Read the model definition and answer for the solid it produces. Units are mm, in the model's axes. A direction names the side the tool comes from. Coordinates: 2 decimals unless noted, no trailing zeros. Order: outer loops, then holes, each group sorted by start corner. A loop starts at its lowest first (then second) coordinate and runs counter-clockwise, first axis right, second up. Notation, with made-up numbers: M 58,6 L 68,6 A22 ccw 68,32 Z; hole C -39.75,-38.75 d11. An arc over 180 degrees is marked long. Put each result on its own line as item: value.
from build123d import *

# Parameters (mm, degrees)
F0_R         = 56.0284560605
F1_DEPTH     = 56.18732
F2_T         = -2.54
F3_W         = 7.7828075737
F3_H         = 34.1701302677
F4_DEPTH     = 276.60562
F6_R         = 34.5946759053
F7_DEPTH     = 25.4
F8_T         = 2.54
F8_T3_DEPTH  = 39.2501302677
F8_T5_DEPTH  = 12.8628075737
F10_SIZE     = 2.54
F11_W        = 6.7604319192
F11_H        = 35.768898204
F12_DEPTH    = 28.2828
F13_W        = 6.7604319192
F13_H        = 35.768898204
F14_DEPTH    = 6.19419
F15_W        = 35.768898204
F15_H        = 8.6004413581
F16_DEPTH    = 43.51639
F17_W        = 31.8477451801
F17_H        = 4.8072040081
F18_DEPTH    = 48.07886
F19_DEPTH    = 32.39902
F20_R        = 5.08
F21_T1_DEPTH = 61.168898204
F22_R        = 1.27


# Not quite as in the source:
# - a fillet or chamfer that OpenCascade refuses, or shapes differently, is made with other operations: its cross-section is extruded or revolved along the edge and cut away or added
# - a shell that OpenCascade refuses in one call is made with other operations: the cavity is built on its own and cut out


with BuildPart() as f1:
    # F0 (on Top) → F1 (new body)
    with BuildSketch(Plane.XY):
        Circle(F0_R)
    extrude(amount=F1_DEPTH)

    # F2
    f2_openings = [f1.faces().sort_by_distance(p)[0] for p in [
        (0, 0, 0),
    ]]
    offset(amount=F2_T, openings=f2_openings)

    # F3 (on face) → F4 (join)
    with BuildSketch(Plane(origin=(0, 0, 53.64732), x_dir=(1, 0, 0), z_dir=(0, 0, -1))):
        with Locations((0.0409056073, 0.1802544365)):
            Rectangle(F3_W, F3_H)
    extrude(amount=F4_DEPTH)

    # F5: chamfer of 5.08 on 1 edges, made by hand

    # F5_s1 → F5_t2 (revolve, cut)
    with BuildSketch(Plane.XZ):
        Polygon((58.5684560605, 0), (53.4884560605, 5.08), (53.4884560605, 0), align=None)
    revolve(axis=Axis((0, 0, 0), (0, 0, 1)), mode=Mode.SUBTRACT)

    # F6 (on face) → F7 (join)
    with BuildSketch(Plane.XY.offset(56.18732)):
        Circle(F6_R)
    extrude(amount=F7_DEPTH)

    # F8: shell of thickness 2.54, made by hand


with BuildPart() as f8_core1:
    # F8_t2: copy of F1
    add(f1.part)

    # the walls: a layer under each face that stays
    f8_faces = [f8_core1.faces().sort_by_distance(p)[0] for p in [
        (-56.0284560605, 0, 29.36366),
        (-54.7584560605, 0, 3.81),
        (-37.3523040403, -37.3523040403, 56.18732),
        (-53.4884560605, 0, 29.36366),
        (-34.5946759053, 0, 68.88732),
        (-35.658970707, -35.658970707, 53.64732),
        (3.9323093942, -0.1802544365, -84.65549),
        (0.0409056073, 16.9048106974, -84.65549),
        (-3.8504981795, -0.1802544365, -84.65549),
        (0.0409056073, -17.2653195703, -84.65549),
    ]]
    thicken(f8_faces, amount=-F8_T, mode=Mode.SUBTRACT)

    # F8_s4 → F8_t3 (cut)
    with BuildSketch(Plane.XZ.offset(-19.4448106974)):
        Polygon((3.9577093942, 53.62192), (3.9323093942, 56.18732), (1.3923093942, 56.18732), (1.3923093942, 53.64732), align=None)
        Polygon((-3.8758981795, 53.62192), (-3.8504981795, 56.18732), (-1.3104981795, 56.18732), (-1.3104981795, 53.64732), align=None)
    extrude(amount=F8_T3_DEPTH, mode=Mode.SUBTRACT)

    # F8_s6 → F8_t5 (cut)
    with BuildSketch(Plane.YZ.offset(-6.3904981795)):
        Polygon((16.9302106974, 53.62192), (16.9048106974, 56.18732), (14.3648106974, 56.18732), (14.3648106974, 53.64732), align=None)
        Polygon((-17.2907195703, 53.62192), (-17.2653195703, 56.18732), (-14.7253195703, 56.18732), (-14.7253195703, 53.64732), align=None)
    extrude(amount=F8_T5_DEPTH, mode=Mode.SUBTRACT)

    # F8_s7 → F8_t8 (revolve, cut)
    with BuildSketch(Plane.XZ):
        Polygon((34.6200759053, 56.21272), (34.5946759053, 53.64732), (32.0546759053, 53.64732), (32.0546759053, 56.18732), align=None)
    revolve(axis=Axis((0, 0, 56.18732), (0, 0, 1)), mode=Mode.SUBTRACT)

    # F8_s9 → F8_t10 (revolve, cut)
    with BuildSketch(Plane.XZ):
        Polygon((53.4630560605, 53.62192), (56.0284560605, 53.64732), (56.0284560605, 56.18732), (53.4884560605, 56.18732), align=None)
    revolve(axis=Axis((0, 0, 53.64732), (0, 0, -1)), mode=Mode.SUBTRACT)


with BuildPart() as f1_1:
    add(f1.part)

    # what is left inside the walls is the cavity
    f8_cavity = [f8_core1.part.solids().sort_by_distance(p)[0] for p in [
        (1.366909, -5.028609, -83.38549),
    ]]
    add(f8_cavity, mode=Mode.SUBTRACT)

    # F9: chamfer of 5.08 on 2 edges, made by hand

    # F9_s1 → F9_t2 (revolve)
    with BuildSketch(Plane.XZ):
        Polygon((39.6746759053, 56.18732), (34.5946759053, 61.26732), (34.5946759053, 56.18732), align=None)
    revolve(axis=Axis((0, 0, 56.18732), (0, 0, 1)))

    # F9_s3 → F9_t4 (revolve, cut)
    with BuildSketch(Plane.XZ):
        Polygon((34.5946759053, 76.50732), (29.5146759053, 81.58732), (34.5946759053, 81.58732), align=None)
    revolve(axis=Axis((0, 0, 81.58732), (0, 0, 1)), mode=Mode.SUBTRACT)

    # F10
    f10_edges = [f1_1.edges().sort_by_distance(p)[0] for p in [
        (-56.028456, 0, 56.18732),
    ]]
    chamfer(f10_edges, length=F10_SIZE)

    # F11 (on face) → F12 (join)
    with BuildSketch(Plane.XY.offset(56.18732)):
        with Locations((0.176892383, -0.2430817112)):
            Rectangle(F11_W, F11_H)
    extrude(amount=F12_DEPTH)

    # F13 (on face) → F14 (join)
    with BuildSketch(Plane.XY.offset(84.47012)):
        with Locations((0.176892383, -0.2430817112)):
            Rectangle(F13_W, F13_H)
    extrude(amount=F14_DEPTH)

    # F15 (on face) → F16 (join)
    with BuildSketch(Plane.YZ.offset(3.5571083426)):
        with Locations((-0.2430817112, 86.3640893209)):
            Rectangle(F15_W, F15_H)
    extrude(amount=F16_DEPTH)

    # F17 (on face) → F18 (cut)
    with BuildSketch(Plane.YZ.offset(47.0734983426)):
        with Locations((0.0361893326, 86.1349776387)):
            Rectangle(F17_W, F17_H)
    extrude(amount=-F18_DEPTH, mode=Mode.SUBTRACT)

    # F19 (cut): a face of the model
    f19_faces = [f1_1.faces().sort_by_distance(p)[0] for p in [
        (0.0409056074, -0.1802544364, 56.18732),
    ]]
    extrude(f19_faces, amount=-F19_DEPTH, mode=Mode.SUBTRACT)

    # F20
    f20_edges = [f1_1.edges().sort_by_distance(p)[0] for p in [
        (-3.203324, -0.243082, 90.66431),
    ]]
    fillet(f20_edges, radius=F20_R)

    # F21: fillet of radius 5.08 on 2 edges, made by hand

    # F21_s2 → F21_t1 (cut)
    with BuildSketch(Plane.XZ.offset(-30.3413673908)):
        with BuildLine():
            ThreePointArc((41.9934983426, 90.66431), (45.5856007911, 89.1764124484), (47.0734983426, 85.58431))
            Line((47.0734983426, 85.58431), (47.0734983426, 90.66431))
            Line((47.0734983426, 90.66431), (41.9934983426, 90.66431))
        make_face()
        with BuildLine():
            ThreePointArc((47.0734983426, 87.1438686419), (45.5856007911, 83.5517661934), (41.9934983426, 82.0638686419))
            Line((41.9934983426, 82.0638686419), (47.0734983426, 82.0638686419))
            Line((47.0734983426, 82.0638686419), (47.0734983426, 87.1438686419))
        make_face()
    extrude(amount=F21_T1_DEPTH, mode=Mode.SUBTRACT)

    # F22
    f22_edges = [f1_1.edges().sort_by_distance(p)[0] for p in [
        (21.935087, -18.127531, 90.66431),
        (21.935087, 17.641367, 90.66431),
        (22.775303, -18.127531, 82.063869),
        (22.775303, 17.641367, 82.063869),
        (3.557108, -18.127531, 69.125594),
        (3.557108, 17.641367, 69.125594),
        (3.932309, 16.904811, -84.65549),
        (3.932309, -17.26532, -84.65549),
        (-3.850498, 16.904811, -84.65549),
        (-3.850498, -17.26532, -84.65549),
    ]]
    fillet(f22_edges, radius=F22_R)


solid = f1_1.part
Q1. Consider line 1 along X through (y, z) = (0, 17); line 2 along Z through (x, y) = (39.5, 11.5); line 3 along Y through (x, z) = (0, 62). Determine where each line is inside the solid, lowest interval first.
Answers below:
line 1: x = -56.03 to -53.49, -3.85 to -1.31, 1.39 to 3.93, 53.49 to 56.03
line 2: z = 53.65 to 56.19, 82.06 to 83.73, 88.54 to 90.66
line 3: y = -34.59 to -32.05, -18.13 to -14.73, 14.36 to 17.64, 32.05 to 34.59
Q2. Given pin 1 (6 mm diameter, centred on x = -1, z = -63, fed in from +Y); pin 2 (12 mm diameter, centred on x = -21, y = -2, fed in from -Z); pin 3 (1.5 mm diameter, centred on y = 3.5, z = -154.5, fed in from +X), each flat-ended and moving along its own axis, determine where each tip first touches the part or whether it passes through.
Answers below:
pin 1: stops at y = 16.9
pin 2: stops at z = 53.65
pin 3: stops at x = 3.93
Q3. For a pull along Z with two mould halves and no side action, classify faces 4 (the face through (-12.146, -54.696, 27.736)), 5 (the face through (-11.622, -52.337, 4.957)), 6 (the face through (23, 0, 88.539)), 7 (the face through (-11.63, -52.37, 56.03)) as +Z half, -Z half, draft (parallel to the pull), parting line (faces both ways), or undercut.
Answers below:
face 4: draft
face 5: -Z half
face 6: undercut
face 7: +Z half
Q4. Find section A-A on z = -60. Write down the section's boundary in (x, y), plus the area to 3 significant figures.
Answers below:
outline: M -3.85,-16 A1.27 ccw -2.58,-17.27 L 2.66,-17.27 A1.27 ccw 3.93,-16 L 3.93,15.63 A1.27 ccw 2.66,16.9 L -2.58,16.9 A1.27 ccw -3.85,15.63 Z; hole M -1.31,-14.73 L 1.39,-14.73 L 1.39,14.36 L -1.31,14.36 Z
area: 186 mm^2
Q5. A tool of negligible diameter and unlimited length cuts with its end or side. For faces 1 (the face through (-27.453, -21.05, 68.781)), 2 (the face through (11, 1, 53.647)), 3 (the face through (23, 0, 82.064)), from which of +Z, -Z, +X, -X, +Y, -Y can it reach the whole face along a straight path? Write none if from no direction.
Answers below:
face 1: none
face 2: -Z
face 3: +X, +Y, -Y
